```python
from build123d import *

# Parameters (mm, degrees)
BOSS_EXTRUDE1_DEPTH  = 5
CHAMFER1_SIZE        = 1
SKETCH2_R            = 1.5
CUT_EXTRUDE1_DEPTH   = 5
LPATTERN1_COUNT      = 2
LPATTERN1_PITCH      = 130
LPATTERN1_COUNT_DIR2 = 2
LPATTERN1_PITCH_DIR2 = 75
SKETCH3_R            = 1.5
CUT_EXTRUDE2_DEPTH   = 5
LPATTERN2_COUNT      = 2
LPATTERN2_PITCH      = 70
LPATTERN3_COUNT      = 2
LPATTERN3_PITCH      = 65


with BuildPart() as part:
    # Sketch1 → Boss-Extrude1 (new body)
    with BuildSketch(Plane(origin=(0, 0, 0), x_dir=(1, 0, 0), z_dir=(0, 1, 0))):
        Polygon((140, 150), (140, 0), (0, 0), (0, 85), (60, 85), (60, 150), align=None)
    extrude(amount=BOSS_EXTRUDE1_DEPTH)

    # Chamfer1
    chamfer1_edges = [part.edges().sort_by_distance(p)[0] for p in [
        (140, 5, -75),
        (100, 5, -150),
        (60, 5, -117.5),
        (30, 5, -85),
        (0, 5, -42.5),
        (70, 5, 0),
    ]]
    chamfer(chamfer1_edges, length=CHAMFER1_SIZE)

    # Sketch2 → Cut-Extrude1 (cut)
    with BuildSketch(Plane(origin=(0, 5, 0), x_dir=(1, 0, 0), z_dir=(0, 1, 0))):
        with Locations((5, 80)):
            Circle(SKETCH2_R)
    cut_extrude1 = extrude(amount=-CUT_EXTRUDE1_DEPTH, mode=Mode.SUBTRACT)

    # LPattern1: Cut-Extrude1 2 × 2
    with Locations(*[(i * LPATTERN1_PITCH, 0, j * LPATTERN1_PITCH_DIR2) for i in range(LPATTERN1_COUNT) for j in range(LPATTERN1_COUNT_DIR2) if (i, j) != (0, 0)]):
        add(cut_extrude1, mode=Mode.SUBTRACT)

    # Sketch3 → Cut-Extrude2 (cut)
    with BuildSketch(Plane(origin=(0, 5, 0), x_dir=(1, 0, 0), z_dir=(0, 1, 0))):
        with Locations((65, 145)):
            Circle(SKETCH3_R)
    cut_extrude2 = extrude(amount=-CUT_EXTRUDE2_DEPTH, mode=Mode.SUBTRACT)

    # LPattern2: Cut-Extrude2 ×2
    with Locations(*[(i * LPATTERN2_PITCH, 0, 0) for i in range(1, LPATTERN2_COUNT)]):
        add(cut_extrude2, mode=Mode.SUBTRACT)

    # LPattern3: Cut-Extrude2 ×2
    with Locations(*[(0, 0, i * LPATTERN3_PITCH) for i in range(1, LPATTERN3_COUNT)]):
        add(cut_extrude2, mode=Mode.SUBTRACT)


solid = part.part
```
Model file for the job. Use its own axes, mm. A direction names the side the tool comes from. Coordinates: 2 decimals unless noted, no trailing zeros. Order: outer loops, then holes, each group sorted by start corner. A loop starts at its lowest first (then second) coordinate and runs counter-clockwise, first axis right, second up. Notation, with made-up numbers: (23.5, -4) - (62.5, -4) arc R20 ccw to (62.5, 27) - close; hole circle Ø6 at (66, -24). An arc over 180 degrees is marked (long way). Return JSON: item names as keys, results as strings. Group by question number.
1) Saw through at B-B, the plane x = 24. Write the cut outline in (y, z), plus the area to 3 significant figures.
2) Saw through at A-A, the plane y = 1.95. Write the cut outline in (x, z).
3) Tool access for faces 1 (the flat face through (60, 2, -117)), 2 (the flat face through (71, 2, 0)): list every direction of +Z, -Z, +X, -X, +Y, -Y with a clear straight run to the whole face (end or side of a thin tool).
4) Saw through at C-C, the plane z = -139. Write the cut outline in (x, y).
5) Flat gauge pins, fed straight in: P1, Ø3, axis at x = 41, y = 2, coming from the -Z side; P2, Ø1.2, axis at y = 1.5, z = -130, coming from the -X side. Where does each tip first touch, or does it go through?
6) Probe line 1 (X direction, y = 1.3, z = -80); line 2 (Z direction, x = 135, y = 3.6); line 3 (X direction, y = 3.8, z = -5). List the from-to ranges inside material, lowest first. Write a range as from..to.
Values found:
{
 "1": {"outline": "(0, -85) - (4, -85) - (5, -84) - (5, -1) - (4, 0) - (0, 0) - close", "area": "424 mm²"},
 "2": {"outline": "(0, -85) - (60, -85) - (60, -150) - (140, -150) - (140, 0) - (0, 0) - close; hole circle Ø3 at (5, -80); hole circle Ø3 at (5, -5); hole circle Ø3 at (65, -145); hole circle Ø3 at (65, -80); hole circle Ø3 at (135, -145); hole circle Ø3 at (135, -80); hole circle Ø3 at (135, -5)"},
 "3": {"face 1": "-Z, -X, +Y, -Y", "face 2": "+Z, +X, -X, +Y, -Y"},
 "4": {"outline": "(60, 0) - (140, 0) - (140, 4) - (139, 5) - (61, 5) - (60, 4) - close"},
 "5": {"P1": "stops at z = -85", "P2": "stops at x = 60"},
 "6": {"line 1": "x = 0..3.5, 6.5..63.5, 66.5..133.5, 136.5..140", "line 2": "z = -150..-146.5, -143.5..-81.5, -78.5..-6.5, -3.5..0", "line 3": "x = 0..3.5, 6.5..133.5, 136.5..140"}
}
